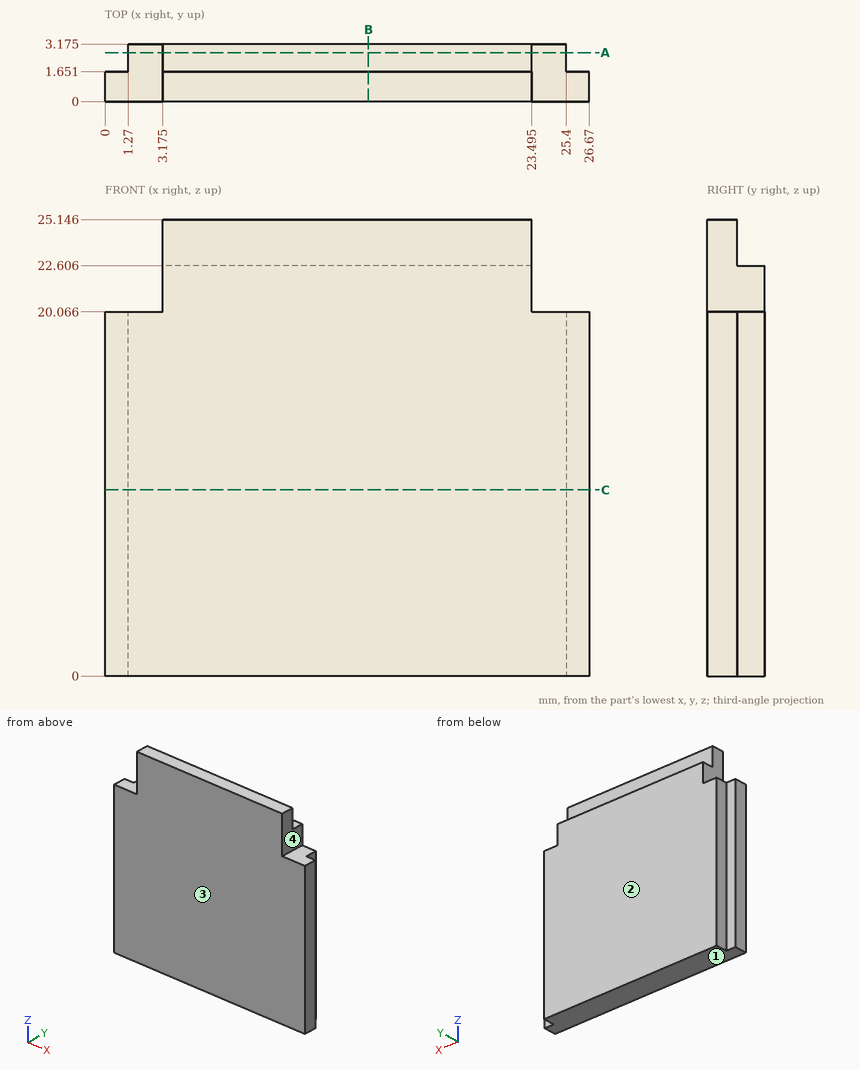
Answer from the drawing. Dimensions are ordinates in mm from the lowest x, y and z of the part. A direction names the side the tool comes from. Coordinates: 2 decimals unless noted, no trailing zeros. Loops run counter-clockwise (first coordinate to the right, second up) from the corner with the lowest first, then second, coordinate; pieces in that order, holes last.
1) Flat-ended cylindrical pins translate along their axes: pin 1 (1 mm diameter, centred on x = 0.5, z = 10, fed in from +Y); pin 2 (0.5 mm diameter, centred on y = 3, z = 12.5, fed in from -X); pin 3 (1.2 mm diameter, centred on x = 12.5, y = 2.5, fed in from +Z). Find the tip coordinate at first contact, or state that the pin passes through.
Results:
pin 1: stops at y = 1.65
pin 2: stops at x = 1.27
pin 3: stops at z = 22.61
2) Section C-C (z = 10.25) is taken. Give the vertices of the cut face in (x, y) (3 decimals).
Results:
outline: (0, 0) - (26.67, 0) - (26.67, 1.651) - (25.4, 1.651) - (25.4, 3.175) - (1.27, 3.175) - (1.27, 1.651) - (0, 1.651) - close
3) Section A-A (y = 2.7) is taken. Give the vertices of the cut face in (x, z) (3 decimals).
Results:
outline: (1.27, 0) - (25.4, 0) - (25.4, 20.066) - (23.495, 20.066) - (23.495, 22.606) - (3.175, 22.606) - (3.175, 20.066) - (1.27, 20.066) - close
4) Consider probe 1 along Z at (x, y) = (1.5, 1.4); probe 2 along X at (y, z) = (1.75, 15.75); probe 3 along Z at (x, y) = (4.5, 2.65). Determine where each line is inside the solid, lowest interval first.
Results:
probe 1: z = 0 to 20.07
probe 2: x = 1.27 to 25.4
probe 3: z = 0 to 22.61
5) Section B-B (x = 14.5) is taken. Give the vertices of the cut face in (y, z) (3 decimals), plus the area to 3 significant figures.
Results:
outline: (0, 0) - (3.175, 0) - (3.175, 22.606) - (1.651, 22.606) - (1.651, 25.146) - (0, 25.146) - close
area: 76.0 mm2
6) For a pull along Z with two mould halves and no side action, classify the marked faces 1 and 2 as +Z half, -Z half, draft (parallel to the pull), parting line (faces both ways), or undercut.
Results:
face 1: -Z half
face 2: draft
7) For the marked faces 3 and 4, determine the directions among +Z, -Z, +X, -X, +Y, -Y from which every point of the face is accessible in a straight line to the end or side of a thin tool.
Results:
face 3: +Z, -Z, +X, -X, -Y
face 4: +Z, +X, +Y, -Y
